```python
from build123d import *

# Parameters (mm, degrees)
SKETCH1_R           = 5
BOSS_EXTRUDE1_DEPTH = 10
SKETCH2_W           = 2
SKETCH2_H           = 30
BOSS_EXTRUDE2_DEPTH = 1


with BuildPart() as part:
    # Sketch1 → Boss-Extrude1 (new, symmetric)
    with BuildSketch(Plane(origin=(0, 0, 0), x_dir=(0, 0, -1), z_dir=(1, 0, 0))):
        Circle(SKETCH1_R)
    extrude(amount=BOSS_EXTRUDE1_DEPTH, both=True)

    # Sketch2 → Boss-Extrude2 (add, symmetric)
    with BuildSketch(Plane.XY):
        with Locations((0, -15)):
            Rectangle(SKETCH2_W, SKETCH2_H)
    extrude(amount=BOSS_EXTRUDE2_DEPTH, both=True)


solid = part.part
```
Geometry check sheet. Reference: the model listing, model coordinates, mm. A direction names the side the tool comes from. Coordinates: 2 decimals unless noted, no trailing zeros. Write each loop counter-clockwise with the first axis right and the second up, starting at its lowest first coordinate (ties: lowest second). Pieces come first, ordered by that corner, then holes. Notation, with made-up numbers: M 36,-32 L 85,-32 A18 ccw 85,-20 Z; hole C 85,35 d1. An arc over 180 degrees is marked long. Answer as a JSON object with one key per item and string values.
1. Scan lines: L1, parallel to Z at x = 0.25, y = -23.5; L2, parallel to Y at x = 6.25, z = 0; L3, parallel to Y at x = -8.75, z = 1. Record each from-to range of solid material in increasing order.
Answers below:
{"L1": "z = -1 to 1", "L2": "y = -5 to 5", "L3": "y = -4.9 to 4.9"}
2. Tool access check on faces 1 (the flat face through (1, -18, 0)), 2 (the flat face through (0, -17, 1)), 3 (the flat face through (0, -17, -1)), 4 (the flat face through (-1, -18, 0)). Record the directions out of +Z, -Z, +X, -X, +Y, -Y that give a thin tool (end or side, any length) a straight path to the whole face; none if there is none.
Answers below:
{"face 1": "+Z, -Z, +X, -Y", "face 2": "+Z, +X, -X, -Y", "face 3": "-Z, +X, -X, -Y", "face 4": "+Z, -Z, -X, -Y"}
3. Section check B-B, the plane y = -13. Enter the section's corners in (x, z), plus the area to 3 significant figures.
Answers below:
{"outline": "M -1,-1 L 1,-1 L 1,1 L -1,1 Z", "area": "4.00 mm²"}
4. Section check A-A, the plane z = 0. Enter the section's corners in (x, y).
Answers below:
{"outline": "M -10,-5 L -1,-5 L -1,-30 L 1,-30 L 1,-5 L 10,-5 L 10,5 L -10,5 Z"}
5. Section check C-C, the plane x = 7.25. Enter the section's corners in (y, z), plus the area to 3 significant figures.
Answers below:
{"outline": "C 0,0 d10", "area": "78.5 mm²"}
6. Go/stop test with flat-tipped pins: pin 1 Ø2 at (x, z) = (0.5, -2.5) entering from -Y; pin 2 Ø6 at (x, y) = (-7, -1) entering from +Z; pin 3 Ø1 at (x, y) = (0, -15.5) entering from +Z; pin 4 Ø2 at (y, z) = (-19.5, 0) entering from -X. Record where each tip stops, or that it passes through.
Answers below:
{"pin 1": "stops at y = -4.77", "pin 2": "stops at z = 5", "pin 3": "stops at z = 1", "pin 4": "stops at x = -1"}
7. Section check D-D, the plane z = 3.5. Enter the section's corners in (x, y).
Answers below:
{"outline": "M -10,-3.57 L 10,-3.57 L 10,3.57 L -10,3.57 Z"}
